Source: three-view drawing plus pictorial views. Frame: mm from the lowest corner of the part. Coordinates: 2 decimals unless noted, no trailing zeros. Loops run counter-clockwise (first coordinate to the right, second up) from the corner with the lowest first, then second, coordinate; pieces in that order, holes last.
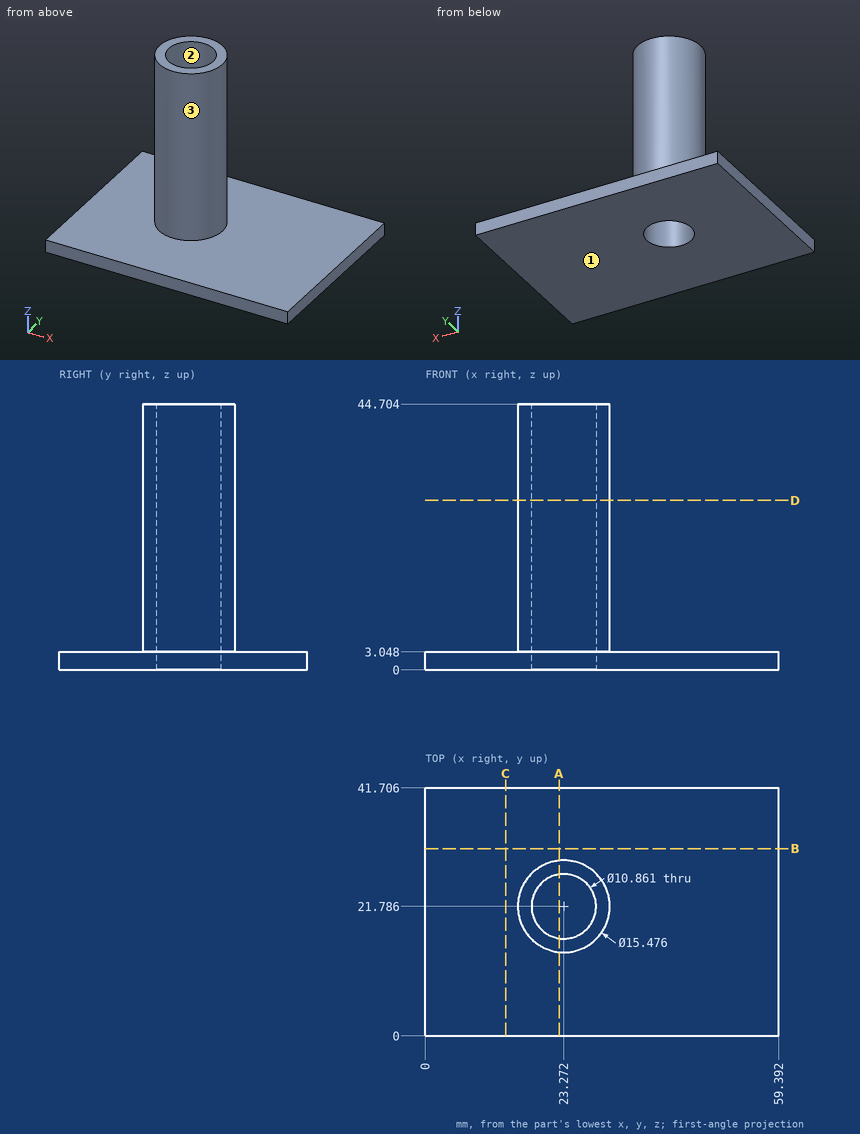
Q1. Section query C-C on x = 13.5. Return the cut outline in (y, z), then the cut area to 3 significant figures.
Q2. Material intervals for line 1 along Y through (x, z) = (23, 34); line 2 along X through (y, z) = (21.5, 34.5) (1 decimal); line 3 along Z through (x, y) = (56.5, 23), sorted ascending.
Q3. First-contact query: pin 1 Ø8 at (y, z) = (21.5, 36.5) entering from -X; pin 2 Ø5 at (y, z) = (21.5, 7) entering from +X; pin 3 Ø5 at (x, z) = (32, 34) entering from -Y (1 decimal). Flat tips, straight axial feed; report the tip coordinate or a pass-through.
Q4. Section query B-B on y = 31.5. Return the cut outline in (x, z), then the cut area to 3 significant figures.
Q5. Section query D-D on z = 28.5. Return the cut outline in (x, y).
Q6. Draft query along X for the marked faces 1, 2 and 3. Return one class per face: released by +X, released by -X, zero draft, split by the parting line, or undercut.
Q7. Section query A-A on x = 22.5. Return the cut outline in (y, z) (1 decimal), then the cut area to 3 significant figures.
Resolved:
1. outline: (0, 0) - (41.71, 0) - (41.71, 3.05) - (0, 3.05) - close
1. area: 127 mm2
2. line 1: y = 14.05 to 16.36, 27.21 to 29.52
2. line 2: x = 15.5 to 17.8, 28.7 to 31
2. line 3: z = 0 to 3.05
3. pin 1: stops at x = 15.53
3. pin 2: stops at x = 31.01
3. pin 3: stops at y = 17.2
4. outline: (0, 0) - (59.39, 0) - (59.39, 3.05) - (0, 3.05) - close
4. area: 181 mm2
5. outline: circle Ø15.48 at (23.27, 21.79); hole circle Ø10.86 at (23.27, 21.79)
6. face 1: zero draft
6. face 2: undercut
6. face 3: split by the parting line
7. outline: (0, 0) - (16.4, 0) - (16.4, 44.7) - (14.1, 44.7) - (14.1, 3) - (0, 3) - close; (27.2, 0) - (41.7, 0) - (41.7, 3) - (29.5, 3) - (29.5, 44.7) - (27.2, 44.7) - close
7. area: 288 mm2
